from build123d import *

# Parameters (mm, degrees)
F0_R     = 19.05
F1_DEPTH = 50.8
F3_DEPTH = 50.8


with BuildPart() as f1:
    # F0 (on Front) → F1 (new body)
    with BuildSketch(Plane.XZ):
        Circle(F0_R)
    extrude(amount=F1_DEPTH)

    # F2 (on face) → F3 (join)
    with BuildSketch(Plane.XZ.offset(50.8)):
        with BuildLine():
            Line((-18.040595, 6.118777), (-13.888012, 3.721282))
            Line((-13.888012, 3.721282), (-10.16673, 10.16673))
            Line((-10.16673, 10.16673), (-14.319314, 12.564225))
            ThreePointArc((-14.319314, 12.564225), (-16.497784, 9.525), (-18.040595, 6.118777))
        make_face()
        with BuildLine():
            Line((-3.721282, 13.888012), (3.721282, 13.888012))
            Line((3.721282, 13.888012), (3.721282, 18.683002))
            ThreePointArc((3.721282, 18.683002), (0, 19.05), (-3.721282, 18.683002))
            Line((-3.721282, 18.683002), (-3.721282, 13.888012))
        make_face()
        with BuildLine():
            Line((10.16673, 10.16673), (13.888012, 3.721282))
            Line((13.888012, 3.721282), (18.040595, 6.118777))
            ThreePointArc((18.040595, 6.118777), (16.497784, 9.525), (14.319314, 12.564225))
            Line((14.319314, 12.564225), (10.16673, 10.16673))
        make_face()
        with BuildLine():
            Line((13.888012, -3.721282), (10.16673, -10.16673))
            Line((10.16673, -10.16673), (14.319314, -12.564225))
            ThreePointArc((14.319314, -12.564225), (16.497784, -9.525), (18.040595, -6.118777))
            Line((18.040595, -6.118777), (13.888012, -3.721282))
        make_face()
        with BuildLine():
            Line((3.721282, -18.683002), (3.721282, -13.888012))
            Line((3.721282, -13.888012), (-3.721282, -13.888012))
            Line((-3.721282, -13.888012), (-3.721282, -18.683002))
            ThreePointArc((-3.721282, -18.683002), (0, -19.05), (3.721282, -18.683002))
        make_face()
        with BuildLine():
            Line((-14.319314, -12.564225), (-10.16673, -10.16673))
            Line((-10.16673, -10.16673), (-13.888012, -3.721282))
            Line((-13.888012, -3.721282), (-18.040595, -6.118777))
            ThreePointArc((-18.040595, -6.118777), (-16.497784, -9.525), (-14.319314, -12.564225))
        make_face()
        Polygon((3.721282, -13.888012), (10.16673, -10.16673), (13.888012, -3.721282), (13.888012, 3.721282), (10.16673, 10.16673), (3.721282, 13.888012), (-3.721282, 13.888012), (-10.16673, 10.16673), (-13.888012, 3.721282), (-13.888012, -3.721282), (-10.16673, -10.16673), (-3.721282, -13.888012), align=None)
    extrude(amount=F3_DEPTH)


solid = f1.part
Geometry: final body of the model. Coordinates: model frame, mm. A direction names the side the tool comes from. Round coordinates to 2 decimals unless told otherwise and drop trailing zeros. Loops run counter-clockwise (first coordinate to the right, second up) from the corner with the lowest first, then second, coordinate; pieces in that order, holes last. Notation, with made-up numbers: M 78,75 L 133,75 A3 cw 133,79 Z; hole C 61,15.5 d1. An arc over 180 degrees is marked long. Put each result on its own line as item: value. Start each with the question number.
(1) Material intervals for line 1 along Z through (x, y) = (-17, -68); line 2 along Z through (x, y) = (0, -15); line 3 along X through (y, z) = (-57.5, -16), sorted ascending. Write a range as [from, to].
(2) Contact query for flat-ended pins moving along their axis: pin 1 Ø2.5 at (y, z) = (-64.5, 16.5) entering from +X; pin 2 Ø8 at (y, z) = (-71, -2) entering from +X; pin 3 Ø10 at (y, z) = (-74.5, -15) entering from -X. Output: stop coordinate, or through.
(3) Section query C-C (y = -16). Return loops of the section in (x, z).
(4) Section query A-A (z = 0). Return loops of the section in (x, y), then the cut area to 3 significant figures.
(5) Section query B-B (y = -62). Return loops of the section in (x, z), then the cut area to 3 significant figures.
(6) Set-up query: faces 1 (the face through (16, -50.8, 0)), 2 (the face through (6.99, -75.84, 12)), 3 (the face through (3.721, -76, 16)), 4 (the face through (12.214, -75.844, -11.349)). Return all of +Z, -Z, +X, -X, +Y, -Y with unobstructed straight access to the full face (end or side cutting, diameter ignored); none if empty.
(7) Draft query along Z for faces 5 (the face through (-12.3, -75.8, -11.4)), 6 (the face through (15.935, -75.844, 4.903)), 7 (the face through (3.721, -76, -16)), 8 (the face through (12.3, -75.8, 11.4)). Return one class per face: +Z half, -Z half, draft (parallel to the pull), parting line (faces both ways), or undercut.
Findings below:
1. line 1: z = [-8.6, -5.52], [5.52, 8.6]
1. line 2: z = [-19.05, 19.05]
1. line 3: x = [-3.72, 3.72]
2. pin 1: stops at x = 3.72
2. pin 2: stops at x = 17.83
2. pin 3: stops at x = -16.21
3. outline: C 0,0 d38.1
4. outline: M -19.05,-50.8 L -13.89,-50.8 L -13.89,-101.6 L 13.89,-101.6 L 13.89,-50.8 L 19.05,-50.8 L 19.05,0 L -19.05,0 Z
4. area: 3,350 mm2
5. outline: M -18.04,-6.12 A19.05 ccw -14.32,-12.56 L -10.17,-10.17 L -3.72,-13.89 L -3.72,-18.68 A19.05 ccw 3.72,-18.68 L 3.72,-13.89 L 10.17,-10.17 L 14.32,-12.56 A19.05 ccw 18.04,-6.12 L 13.89,-3.72 L 13.89,3.72 L 18.04,6.12 A19.05 ccw 14.32,12.56 L 10.17,10.17 L 3.72,13.89 L 3.72,18.68 A19.05 ccw -3.72,18.68 L -3.72,13.89 L -10.17,10.17 L -14.32,12.56 A19.05 ccw -18.04,6.12 L -13.89,3.72 L -13.89,-3.72 Z
5. area: 845 mm2
6. face 1: +X, -Y
6. face 2: +Z, -Y
6. face 3: +Z, +X, -Y
6. face 4: -Z, -Y
7. face 5: -Z half
7. face 6: undercut
7. face 7: draft
7. face 8: +Z half
